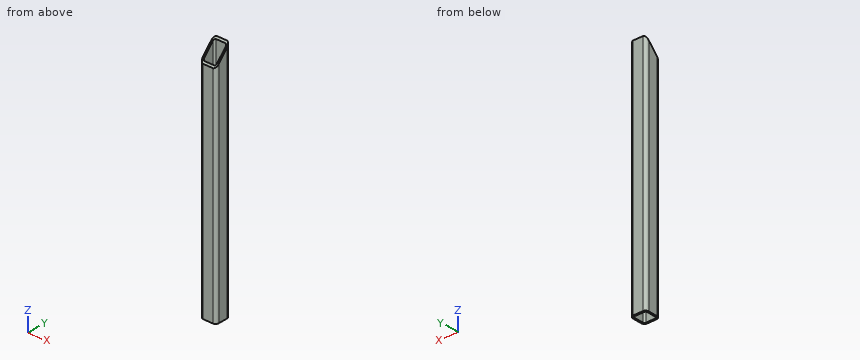
Autodesk Inventor part; units mm, degrees
ref_plane "Start Plane" through (0, 0, 20) normal (0, 0, 1) x (1, 0, 0)
ref_plane "End Plane" through (0, 0, 619.9668) normal (0, 0, 1) x (1, 0, 0)
ref_plane "Work Plane4" through (0, 20.7311, 620.7502) normal (0, -0.7311, 0.6823) x (1, 0, 0)
ref_plane "Start Plane" through (0, 0, 20) normal (0, 0, 1) x (1, 0, 0)
ref_plane "End Plane" through (0, 0, 619.9668) normal (0, 0, 1) x (1, 0, 0)
sketch "Sketch" plane through (0, 0, 0) normal (0, 0, 1) x (1, 0, 0)
  line L0 (-20, -12) -> (-20, 12)
  line L1 (-12, 20) -> (12, 20)
  line L2 (20, 12) -> (20, -12)
  line L3 (12, -20) -> (-12, -20)
  arc A0 (-20, -12) -> (-12, -20) centre (-12, -12) ccw
  arc A1 (20, 12) -> (12, 20) centre (12, 12) ccw
  arc A2 (-12, 20) -> (-20, 12) centre (-12, 12) ccw
  arc A3 (12, -20) -> (20, -12) centre (12, -12) ccw
  arc A4 (-12, 16) -> (-16, 12) centre (-12, 12) ccw
  line L4 (-12, 16) -> (12, 16)
  arc A5 (16, 12) -> (12, 16) centre (12, 12) ccw
  line L5 (16, 12) -> (16, -12)
  arc A6 (12, -16) -> (16, -12) centre (12, -12) ccw
  line L6 (12, -16) -> (-12, -16)
  arc A7 (-16, -12) -> (-12, -16) centre (-12, -12) ccw
  line L7 (-16, -12) -> (-16, 12)
  line L8 (0, 30.3196) -> (0, -30.3196) construction
  line L9 (-30.3196, 0) -> (30.3196, 0) construction
  dimension "d7" = 8
  dimension "d9" = 40
  dimension "d11" = 40
  dimension "d12" = 4
  dimension "d15" = 20
  dimension "d16" = 20
extrude "Body" add sketch "Sketch" along normal up to surface (599.9668 mm away) from surface at 20
sketch "Sketch3" plane through (0, 0, 0) normal (0, 0, 1) x (1, 0, 0)
  line L0 (0, 0) -> (10, 0)
ref_plane "Work Plane3" through (0, 0, 0) normal (0, -1, 0) x (1, 0, 0)
ref_plane "Work Plane4" through (0, 20.7311, 620.7502) normal (0, -0.7311, 0.6823) x (1, 0, 0)
split "Split1" plane through (0, 20.7311, 620.7502) removes the side toward (0, -0.7311, 0.6823)
ref_plane "Work Plane5" through (-12, 0, 20) normal (0, 0, -1) x (-1, 0, 0)
split "Split2" plane through (-12, 0, 20) removes the side toward (0, 0, -1)
sketch "Sketch4" plane through (0, 0, 0) normal (0, -1, 0) x (1, 0, 0)
  line L0 (-2, 20) -> (12, 20)
  line L1 (-2, 619.9668) -> (12, 619.9668)
  dimension "d18" = 599.9668
equation "\"d7\" = G_IR"
equation "\"d9\" = G_W"
equation "\"d11\" = G_H"
equation "\"d12\" = G_T"
equation "\"d15\" = 0.5 * d9"
equation "\"d16\" = 0.5 * d11"
equation "\"d3\" = G_L"
equation "\"G_W\" = 40"
equation "\"G_H\" = 40"
equation "\"G_T\" = 4"
equation "\"G_IR\" = 8"
equation "\"G_L\" = d18"
equation "\"G_OFFSET_END\" = 19.96675"
equation "\"d14\" = G_OFFSET_END + B_L"
properties part number "ISO 10799-2 - 40x40x4 - 599,97" material "Steel, Mild"
Geometry: final body of the model. Coordinates: model frame, mm. Coordinates: 2 decimals unless noted, no trailing zeros. Order: outer loops, then holes, each group sorted by start corner. A loop starts at its lowest first (then second) coordinate and runs counter-clockwise, first axis right, second up. Notation, with made-up numbers: (-19.5, 23) - (8.5, 23) arc R31 ccw to (8.5, 49) - close; hole circle Ø2 at (57, -36.5). An arc over 180 degrees is marked (long way). Return JSON: item names as keys, results as strings. Group by question number.
1. Cut plane B-B (z = 323.5). Output: boundary loops of the cut face in (x, y).
2. Pin query (flat end, axial travel): pin 1 (1 mm diameter, centred on x = 14, z = 555.5, fed in from +Y). Return the tip coordinate at first contact, or that it passes through.
3. Material intervals for line 1 along X through (y, z) = (9, 246); line 2 along X through (y, z) = (-13, 234.5), sorted ascending. Write a range as [from, to].
4. Cut plane C-C (y = -4). Output: boundary loops of the cut face in (x, z), plus the area to 3 significant figures.
5. Cut plane A-A (x = 0). Output: boundary loops of the cut face in (y, z), plus the area to 3 significant figures.
Resolved:
{
 "1": {"outline": "(-20, -12) arc R8 ccw to (-12, -20) - (12, -20) arc R8 ccw to (20, -12) - (20, 12) arc R8 ccw to (12, 20) - (-12, 20) arc R8 ccw to (-20, 12) - close; hole (-16, -12) arc R4 ccw to (-12, -16) - (12, -16) arc R4 ccw to (16, -12) - (16, 12) arc R4 ccw to (12, 16) - (-12, 16) arc R4 ccw to (-16, 12) - close"},
 "2": {"pin 1": "stops at y = 19.86"},
 "3": {"line 1": "x = [-20, -16], [16, 20]", "line 2": "x = [-19.94, -15.87], [15.87, 19.94]"},
 "4": {"outline": "(-20, 20) - (-16, 20) - (-16, 594.25) - (-20, 594.25) - close; (16, 20) - (20, 20) - (20, 594.25) - (16, 594.25) - close", "area": "4,590 mm²"},
 "5": {"outline": "(-20, 20) - (-16, 20) - (-16, 581.39) - (-20, 577.11) - close; (16, 20) - (20, 20) - (20, 619.97) - (16, 615.68) - close", "area": "4,630 mm²"}
}
